Input: part model. Units: mm. Frame: model coordinates. Face numbers are marked on the shaded views. A direction names the side the tool comes from. Round coordinates to 2 decimals unless told otherwise and drop trailing zeros. Order: outer loops, then holes, each group sorted by start corner. A loop starts at its lowest first (then second) coordinate and runs counter-clockwise, first axis right, second up. Notation, with made-up numbers: (-32.75, 44) -> (4.25, 44) arc R26 cw to (4.25, 73) -> close; hole circle Ø1 at (-37.75, 81). An arc over 180 degrees is marked (long way). Use a Markdown table: item, result.
from build123d import *

# Parameters (mm, degrees)
F0_R     = 28.575
F1_DEPTH = 40.2336
F3_DEPTH = 15.7734
F5_DEPTH = 40.2346
F6_R     = 10.16
F7_DEPTH = 15.7744
F8_R     = 3.302


with BuildPart() as f1:
    # F0 (on Top) → F1 (new body)
    with BuildSketch(Plane.XY):
        Circle(F0_R)
    extrude(amount=F1_DEPTH)

    # F2 (on Top) → F3 (join)
    with BuildSketch(Plane.XY):
        with BuildLine():
            Line((5.042647, -28.126541), (57.336765, -18.751028))
            ThreePointArc((57.336765, -18.751028), (73.025, 0), (57.336765, 18.751028))
            Line((57.336765, 18.751028), (5.042647, 28.126541))
            ThreePointArc((5.042647, 28.126541), (-28.575, 0), (5.042647, -28.126541))
        make_face()
    extrude(amount=F3_DEPTH)

    # F4 (on face) → F5 (cut, through all)
    with BuildSketch(Plane.XY.offset(40.2336)):
        with BuildLine():
            Line((18.5293, 4.064), (13.697319, 4.064))
            ThreePointArc((13.697319, 4.064), (-14.2875, 0), (13.697319, -4.064))
            Line((13.697319, -4.064), (18.5293, -4.064))
            Line((18.5293, -4.064), (18.5293, 0))
            Line((18.5293, 0), (18.5293, 4.064))
        make_face()
    extrude(amount=-F5_DEPTH, mode=Mode.SUBTRACT)

    # F6 (on face) → F7 (cut, through all)
    with BuildSketch(Plane.XY.offset(15.7734)):
        with Locations((53.975, 0)):
            Circle(F6_R)
    extrude(amount=-F7_DEPTH, mode=Mode.SUBTRACT)

    # F8
    f8_edges = [f1.edges().sort_by_distance(p)[0] for p in [
        (-28.575, 0, 40.2336),
    ]]
    fillet(f8_edges, radius=F8_R)


solid = f1.part
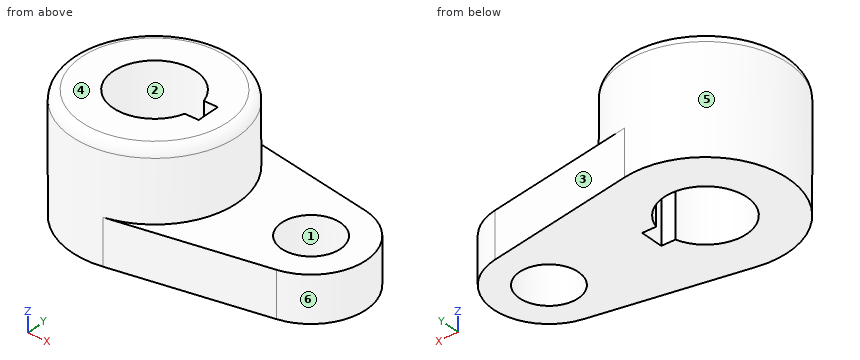
1) Pull-direction query (Y, two-part tool) for the marked faces 1, 2, 3 and 4; classes: +Y half, -Y half, draft (parallel to the pull), parting line (faces both ways), or undercut.
Results found:
| item | result |
|---|---|
| face 1 | undercut |
| face 2 | undercut |
| face 3 | +Y half |
| face 4 | draft |
2) Line query: L1, parallel to X at y = 0, z = 27.5 (1 decimal); L2, parallel to Z at x = 37.5, y = 21; L3, parallel to X at y = 10.5, z = 27.5. Output: solid intervals per line, ascending. Write a range as [from, to].
Results found:
| item | result |
|---|---|
| L1 | x = [-28.6, -14.3], [18.5, 28.6] |
| L2 | z = [0, 15.77] |
| L3 | x = [-26.58, -9.69], [9.69, 26.58] |
3) Cut plane D-D on x = 0. Return loops of the section in (y, z) (1 decimal).
Results found:
| item | result |
|---|---|
| outline | (-28.6, 0) -> (-14.3, 0) -> (-14.3, 40.2) -> (-25.3, 40.2) arc R3.3 ccw to (-28.6, 36.9) -> close; (14.3, 0) -> (28.6, 0) -> (28.6, 36.9) arc R3.3 ccw to (25.3, 40.2) -> (14.3, 40.2) -> close |
4) Set-up query: the marked faces 5 and 6. Return all of +Z, -Z, +X, -X, +Y, -Y with unobstructed straight access to the full face (end or side cutting, diameter ignored); none if empty.
Results found:
| item | result |
|---|---|
| face 5 | +Z |
| face 6 | +Z, -Z, +X |
5) Pin query (flat end, axial travel): pin 1 Ø2 at (y, z) = (-5.5, 27.5) entering from +X; pin 2 Ø5 at (x, y) = (41.5, -17) entering from +Z; pin 3 Ø1 at (x, z) = (-3, 10.5) entering from +Y. Return the tip coordinate at first contact, or that it passes through.
Results found:
| item | result |
|---|---|
| pin 1 | stops at x = 28.22 |
| pin 2 | stops at z = 15.77 |
| pin 3 | stops at y = 28.47 |
6) Cut plane C-C on x = 63. Return loops of the section in (y, z), and give its area (3 significant figures).
Results found:
| item | result |
|---|---|
| outline | (-16.78, 0) -> (-4.67, 0) -> (-4.67, 15.77) -> (-16.78, 15.77) -> close; (4.67, 0) -> (16.78, 0) -> (16.78, 15.77) -> (4.67, 15.77) -> close |
| area | 382 mm² |
7) Cut plane A-A on y = 0. Return loops of the section in (x, z) (1 decimal).
Results found:
| item | result |
|---|---|
| outline | (-28.6, 0) -> (-14.3, 0) -> (-14.3, 40.2) -> (-25.3, 40.2) arc R3.3 ccw to (-28.6, 36.9) -> close; (18.5, 0) -> (43.8, 0) -> (43.8, 15.8) -> (28.6, 15.8) -> (28.6, 36.9) arc R3.3 ccw to (25.3, 40.2) -> (18.5, 40.2) -> close; (64.1, 0) -> (73, 0) -> (73, 15.8) -> (64.1, 15.8) -> close |
